```python
from build123d import *

# Parameters (mm, degrees)
F1_DEPTH = 1371.6
F2_R     = 4.7625
F3_DEPTH = 38.101


with BuildPart() as f1:
    # F0 (on Top) → F1 (new body)
    with BuildSketch(Plane.XY):
        Polygon((0, 3.175), (0, 0), (38.1, 0), (38.1, 38.1), (34.925, 38.1), (34.925, 3.175), align=None)
    extrude(amount=F1_DEPTH)

    # F2 (on face) → F3 (cut, through all)
    with BuildSketch(Plane.XZ):
        with Locations((15.24, 254)):
            Circle(F2_R)
        with Locations((15.24, 558.8)):
            Circle(F2_R)
        with Locations((15.24, 1270)):
            Circle(F2_R)
    extrude(amount=-F3_DEPTH, mode=Mode.SUBTRACT)


solid = f1.part
```
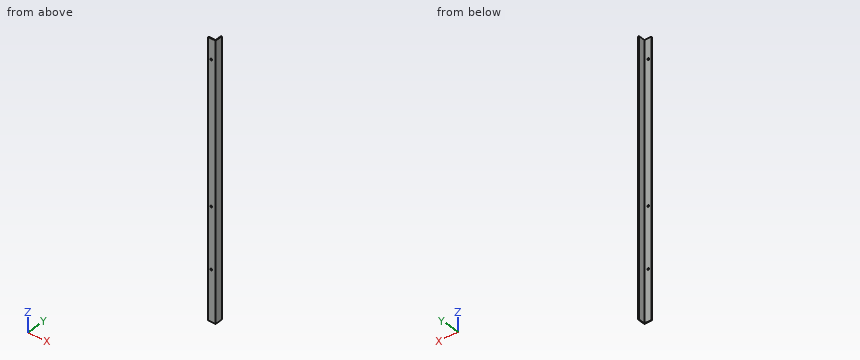
Here's how the part is built. I have some questions about the finished solid (model axes, mm). Coordinates: 2 decimals unless noted, no trailing zeros. Order: outer loops, then holes, each group sorted by start corner. A loop starts at its lowest first (then second) coordinate and runs counter-clockwise, first axis right, second up.
Item 1: I need wall thicknesses on probe 1 along Z at (x, y) = (15, 1); probe 2 along X at (y, z) = (0.95, 1270); probe 3 along X at (y, z) = (18, 1278) (3 decimals). Which ranges of each line are inside material? Lowest first, please.
Response values:
probe 1: z = 0 to 249.24, 258.76 to 554.04, 563.56 to 1265.24, 1274.76 to 1371.6
probe 2: x = 0 to 10.48, 20 to 38.1
probe 3: x = 34.925 to 38.1
Item 2: I'm going to push flat-ended pins straight in: pin 1 Ø15 at (x, z) = (15.24, 254) entering from +Y (3 decimals); pin 2 Ø2 at (y, z) = (23.5, 287) entering from -X (3 decimals); pin 3 Ø10 at (x, y) = (19, 9) entering from -Z. Where does each tip first touch, or does it pass through?
Response values:
pin 1: stops at y = 3.175
pin 2: stops at x = 34.925
pin 3: passes through
Item 3: If we section it at C-C, the plane x = 27: List the corners of the cut face in (y, z) for me (3 decimals).
Response values:
outline: (0, 0) - (3.175, 0) - (3.175, 1371.6) - (0, 1371.6) - close
Item 4: If we section it at B-B, the plane y = 28.5: List the corners of the cut face in (x, z) for me (3 decimals).
Response values:
outline: (34.925, 0) - (38.1, 0) - (38.1, 1371.6) - (34.925, 1371.6) - close
Item 5: If we section it at A-A, the plane z = 1011.5: List the corners of the cut face in (x, y) for me (3 decimals).
Response values:
outline: (0, 0) - (38.1, 0) - (38.1, 38.1) - (34.925, 38.1) - (34.925, 3.175) - (0, 3.175) - close
